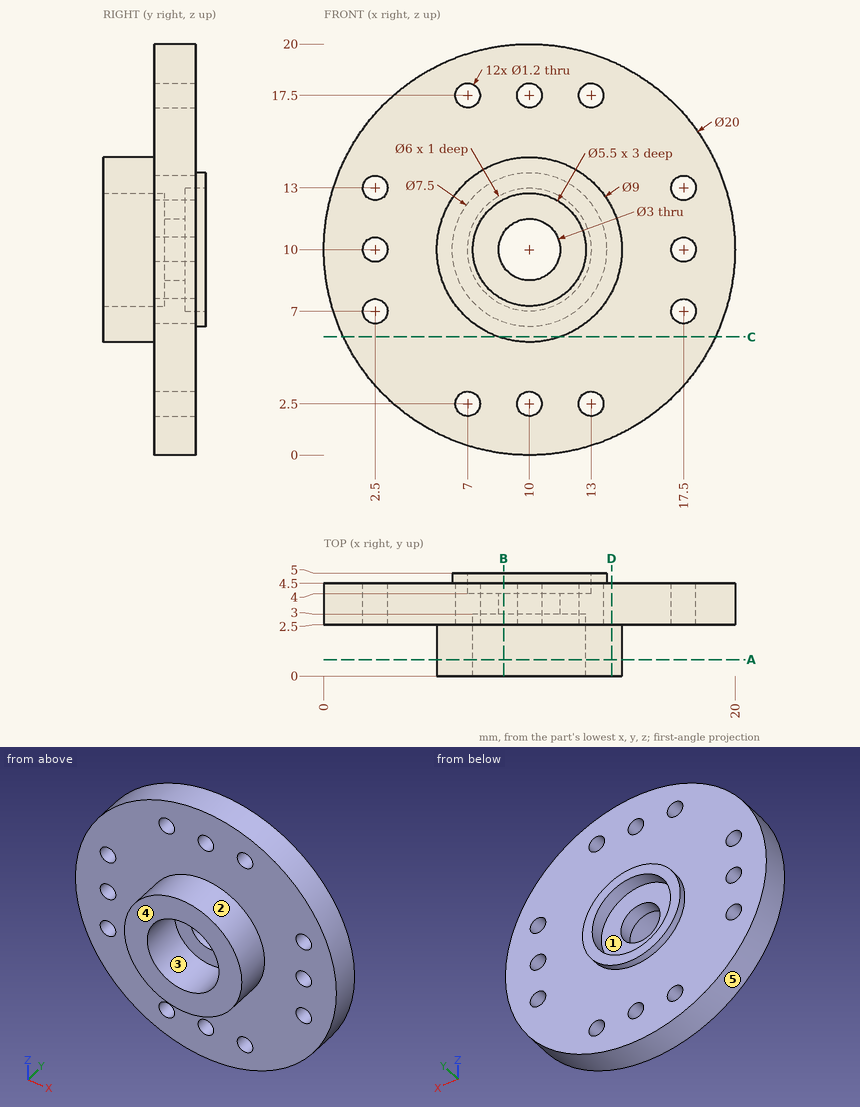
Can you work these out from the drawing? Everything is in mm from the part's minimum corner. A direction names the side the tool comes from. Give positions to 0.01 mm unless a question says otherwise; leave off trailing zeros. Write each loop counter-clockwise with the first axis right and the second up, starting at its lowest first coordinate (ties: lowest second). Pieces come first, ordered by that corner, then holes. Notation, with made-up numbers: M 3.25,43 L 46.25,43 A20 cw 46.25,55 Z; hole C 73,55 d10. An arc over 180 degrees is marked long. Answer in a Markdown table with one row per item. Add a question column.
Item 1: On a 3-axis mill with a long thin cutter (end or side, diameter ignored), from which of +Z, -Z, +X, -X, +Y, -Y can I reach the whole of each face in a straight line? I mean the marked faces 1 and 2. Say none if no direction works.
Item 2: Please list where these lines run through material, in increasing order: L1, parallel to X at y = 3.9, z = 10; L2, parallel to Z at x = 10, y = 4.05; L3, parallel to X at y = 0.4, z = 10.
Item 3: Imagine slicing it at C-C, the plane z = 5.75. Write out the boundary of the cut face in (x, y), plus the area to 3 significant figures.
Item 4: For pin 1 Ø1.6 at (x, z) = (7, 2.5) entering from -Y; pin 2 Ø5 at (x, z) = (10, 10) entering from -Y; pin 3 Ø1.9 at (x, z) = (10, 17.5) entering from +Y; pin 4 Ø1.5 at (x, z) = (8, 8) entering from -Y, each with a flat end and sliding along its axis, tell me the tip position at first contact or that it passes through.
Item 5: We'd pull the mould along Z, two halves only. Please class the marked faces 3, 4 and 5: released by +Z, released by -Z, zero draft, split by the parting line, or undercut.
Item 6: Imagine slicing it at D-D, the plane x = 14. Write out the boundary of the cut face in (y, z).
Item 7: Imagine slicing it at A-A, the plane y = 0.8. Write out the boundary of the cut face in (x, z), plus the area to 3 significant figures.
Item 8: Imagine slicing it at B-B, the plane x = 8.75. Write out the boundary of the cut face in (y, z).
Evaluation:
| question | item | result |
|---|---|---|
| 1 | face 1 | +Y |
| 1 | face 2 | -Y |
| 2 | L1 | x = 0 to 1.9, 3.1 to 8.5, 11.5 to 16.9, 18.1 to 20 |
| 2 | L2 | z = 0 to 1.9, 3.1 to 7, 13 to 16.9, 18.1 to 20 |
| 2 | L3 | x = 5.5 to 7.25, 12.75 to 14.5 |
| 3 | outline | M 0.95,2.5 L 8.52,2.5 L 8.52,0 L 11.48,0 L 11.48,2.5 L 19.05,2.5 L 19.05,4.5 L 0.95,4.5 Z |
| 3 | area | 43.6 mm² |
| 4 | pin 1 | stops at y = 2.5 |
| 4 | pin 2 | stops at y = 3 |
| 4 | pin 3 | stops at y = 4.5 |
| 4 | pin 4 | stops at y = 0 |
| 5 | face 3 | undercut |
| 5 | face 4 | zero draft |
| 5 | face 5 | split by the parting line |
| 6 | outline | M 0,7.94 L 2.5,7.94 L 2.5,0.83 L 4.5,0.83 L 4.5,19.17 L 2.5,19.17 L 2.5,12.06 L 0,12.06 Z |
| 7 | outline | C 10,10 d9; hole C 10,10 d5.5 |
| 7 | area | 39.9 mm² |
| 8 | outline | M 0,5.68 L 2.5,5.68 L 2.5,0.08 L 4.5,0.08 L 4.5,6.46 L 5,6.46 L 5,7.27 L 4,7.27 L 4,9.17 L 3,9.17 L 3,7.55 L 0,7.55 Z; M 0,12.45 L 3,12.45 L 3,10.83 L 4,10.83 L 4,12.73 L 5,12.73 L 5,13.54 L 4.5,13.54 L 4.5,19.92 L 2.5,19.92 L 2.5,14.32 L 0,14.32 Z |
